Input: part model. Units: mm. Frame: model coordinates. Face numbers are marked on the shaded views. A direction names the side the tool comes from. Round coordinates to 2 decimals unless told otherwise and drop trailing zeros. Order: outer loops, then holes, each group sorted by start corner. A loop starts at its lowest first (then second) coordinate and runs counter-clockwise, first axis right, second up. Notation, with made-up numbers: (72.25, 59.25) -> (117.25, 59.25) arc R26 ccw to (117.25, 81.25) -> close; hole circle Ø9 at (45.5, -36.5). An arc over 180 degrees is marked (long way). Use a Markdown table: item, result.
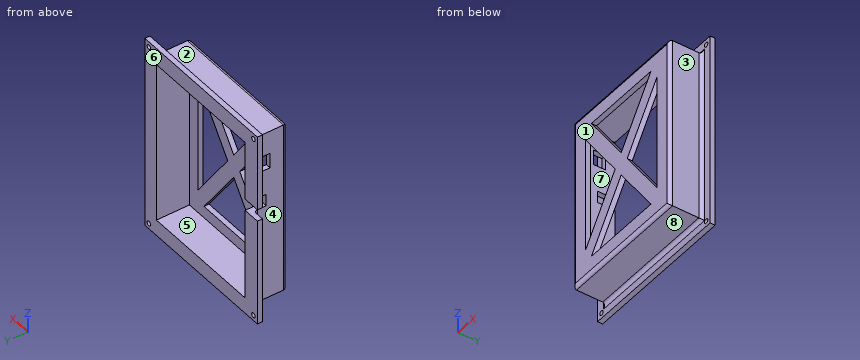
from build123d import *

# Parameters (mm, degrees)
SKETCH1_W              = 72.5
SKETCH1_H              = 96.5
BRACKETBASE_DEPTH      = 3
SKETCH3_W              = 78.5
SKETCH3_H              = 102.5
SKETCH3_W_2            = 72.5
SKETCH3_H_2            = 96.5
BRACKETWALLS_DEPTH     = 22.5
SKETCH4_W              = 7
SKETCH4_H              = 19.5
WIREHOLE_DEPTH         = 22.5
BRACKETFLANGE_DEPTH    = 3
SKETCH7_R              = 1.375
MOUNTINGHOLES_DEPTH    = 4
SKETCH8_W              = 9
SKETCH8_H              = 7
SWITCHHOLE_DEPTH       = 10
BOSS_EXTRUDE1_REACH    = 72.85
SKETCH10_W             = 2.5
SKETCH10_H             = 7
BOSS_EXTRUDE2_DEPTH    = 12.25
FILLET1_R              = 2
FILLET2_R              = 2
SKETCH11_W             = 7
SKETCH11_H             = 10.25
CUT_EXTRUDE1_DEPTH     = 10
WEIGHTREDUCTION1_DEPTH = 23.5


with BuildPart() as part:
    # Sketch1 → bracketBase (new body)
    with BuildSketch(Plane(origin=(0, 0, 0), x_dir=(1, 0, 0), z_dir=(0, 1, 0))):
        with Locations((36.25, 48.25)):
            Rectangle(SKETCH1_W, SKETCH1_H)
    extrude(amount=BRACKETBASE_DEPTH)

    # Sketch3 → bracketWalls (add)
    with BuildSketch(Plane.XZ):
        with Locations((36.25, -48.25)):
            Rectangle(SKETCH3_W, SKETCH3_H)
        with Locations((36.25, -48.25)):
            Rectangle(SKETCH3_W_2, SKETCH3_H_2, mode=Mode.SUBTRACT)
    extrude(amount=-BRACKETWALLS_DEPTH)

    # Sketch4 → wireHole (cut)
    with BuildSketch(Plane.ZY.offset(-72.5)):
        with Locations((-38.65, 12.75)):
            Rectangle(SKETCH4_W, SKETCH4_H)
    wirehole = extrude(amount=-WIREHOLE_DEPTH, mode=Mode.SUBTRACT)

    # Sketch6 → bracketFlange (add)
    with BuildSketch(Plane(origin=(0, 22.5, 0), x_dir=(1, 0, 0), z_dir=(0, 1, 0))):
        Polygon((72.5, 96.5), (72.5, 42.15), (82, 42.15), (82, 106), (-10, 106), (-10, -10), (82, -10), (82, 35.15), (72.5, 35.15), (72.5, 0), (0, 0), (0, 96.5), align=None)
    extrude(amount=-BRACKETFLANGE_DEPTH)

    # Sketch7 → mountingHoles (cut, through all)
    with BuildSketch(Plane.XZ.offset(-19.5)):
        with Locations((78.75, -102.75)):
            Circle(SKETCH7_R)
        with Locations((78.75, 6.75)):
            Circle(SKETCH7_R)
        with Locations((-6.75, -102.75)):
            Circle(SKETCH7_R)
        with Locations((-6.75, 6.75)):
            Circle(SKETCH7_R)
    extrude(amount=-MOUNTINGHOLES_DEPTH, mode=Mode.SUBTRACT)

    # Mirror1: wireHole across plane
    add(wirehole.mirror(Plane(origin=(36, 0, 0), x_dir=(0, 0, 1), z_dir=(1, 0, 0))), mode=Mode.SUBTRACT)

    # Sketch8 → switchHole (cut)
    with BuildSketch(Plane.ZY.offset(3)):
        with Locations((-15.23, 13.5)):
            Rectangle(SKETCH8_W, SKETCH8_H)
    extrude(amount=-SWITCHHOLE_DEPTH, mode=Mode.SUBTRACT)

    # Sketch9 → Boss-Extrude1 (add, up to next)
    with BuildSketch(Plane(origin=(0, 0, -35.15), x_dir=(-1, 0, 0), z_dir=(0, 0, -1)), mode=Mode.PRIVATE) as boss_extrude1_sk1:
        Polygon((-72.5, 3), (-72.5, 22.5), (-82, 22.5), (-82, 19.5), (-75.5, 19.5), (-75.5, 3), align=None)
    boss_extrude1_tool1 = extrude(boss_extrude1_sk1.sketch, amount=BOSS_EXTRUDE1_REACH, mode=Mode.PRIVATE) - part.part
    add(boss_extrude1_tool1.solids().sort_by_distance((75.1875, 14.8125, -35.15))[0])

    # Sketch10 → Boss-Extrude2 (add)
    with BuildSketch(Plane.XZ):
        with Locations((-1.75, -38.65)):
            Rectangle(SKETCH10_W, SKETCH10_H)
    extrude(amount=-BOSS_EXTRUDE2_DEPTH)

    # Fillet1
    fillet1_edges = [part.edges().sort_by_distance(p)[0] for p in [
        (-3, 19.5, -16.075),
        (36.25, 19.5, 3),
        (75.5, 19.5, -48.25),
        (36.25, 19.5, -99.5),
        (-3, 19.5, -70.825),
    ]]
    fillet(fillet1_edges, radius=FILLET1_R)

    # Fillet2
    fillet2_edges = [part.edges().sort_by_distance(p)[0] for p in [
        (36.25, 0, 3),
        (-3, 0, -48.25),
        (36.25, 0, -99.5),
        (75.5, 0, -48.25),
    ]]
    fillet(fillet2_edges, radius=FILLET2_R)

    # Sketch11 → Cut-Extrude1 (cut)
    with BuildSketch(Plane.ZY.offset(0.5)):
        with Locations((-38.65, 17.375)):
            Rectangle(SKETCH11_W, SKETCH11_H)
    extrude(amount=-CUT_EXTRUDE1_DEPTH, mode=Mode.SUBTRACT)

    # Sketch12 → weightReduction1 (cut, through all)
    with BuildSketch(Plane.XZ):
        Polygon((11.903565914, -89.5), (36.25, -55.165285264), (60.596434086, -89.5), align=None)
        Polygon((65.5, -82.584714736), (41.153565914, -48.25), (65.5, -13.915285264), align=None)
        Polygon((60.596434086, -7), (11.903565914, -7), (36.25, -41.334714736), align=None)
        Polygon((7, -13.915285264), (7, -82.584714736), (31.346434086, -48.25), align=None)
    extrude(amount=-WEIGHTREDUCTION1_DEPTH, mode=Mode.SUBTRACT)


solid = part.part
1) Cut plane D-D on z = 6.75. Return loops of the section in (x, y) (3 decimals).
Answer key:
| item | result |
|---|---|
| outline | (-10, 19.5) -> (-8.125, 19.5) -> (-8.125, 22.5) -> (-10, 22.5) -> close; (-5.375, 19.5) -> (77.375, 19.5) -> (77.375, 22.5) -> (-5.375, 22.5) -> close; (80.125, 19.5) -> (82, 19.5) -> (82, 22.5) -> (80.125, 22.5) -> close |
2) Draft query along Z for the marked faces 6, 7 and 8. Return one class per face: released by +Z, released by -Z, zero draft, split by the parting line, or undercut.
Answer key:
| item | result |
|---|---|
| face 6 | zero draft |
| face 7 | undercut |
| face 8 | released by -Z |
3) Cut plane B-B on y = 4.5. Return loops of the section in (x, z).
Answer key:
| item | result |
|---|---|
| outline | (-3, -99.5) -> (75.5, -99.5) -> (75.5, 3) -> (-3, 3) -> close; hole (0, -96.5) -> (72.5, -96.5) -> (72.5, 0) -> (0, 0) -> close |
4) Set-up query: the marked faces 1, 2, 3, 4 and 5. Return all of +Z, -Z, +X, -X, +Y, -Y with unobstructed straight access to the full face (end or side cutting, diameter ignored); none if empty.
Answer key:
| item | result |
|---|---|
| face 1 | +Z, -Z, +X, -X, -Y |
| face 2 | +Z, +X, -X, -Y |
| face 3 | +Z, -Z, +X, -Y |
| face 4 | +Z, -Z, -X, -Y |
| face 5 | +Y |
5) Ray query, probe 1 along Z at (x, y) = (78.75, 21.85) (3 decimals); probe 2 along Z at (x, y) = (-6.75, 21.3) (3 decimals); probe 3 along X at (y, z) = (12.75, -4). Return the intervals inside material, ascending.
Answer key:
| item | result |
|---|---|
| probe 1 | z = -106 to -104.125, -101.375 to 5.375, 8.125 to 10 |
| probe 2 | z = -106 to -104.125, -101.375 to -42.15, -35.15 to 5.375, 8.125 to 10 |
| probe 3 | x = -3 to 0, 72.5 to 75.5 |
6) Cut plane C-C on x = -6.75. Return loops of the section in (y, z) (3 decimals), and give its area (4 significant figures).
Answer key:
| item | result |
|---|---|
| outline | (19.5, -106) -> (22.5, -106) -> (22.5, -104.125) -> (19.5, -104.125) -> close; (19.5, -101.375) -> (22.5, -101.375) -> (22.5, -42.15) -> (19.5, -42.15) -> close; (19.5, -35.15) -> (22.5, -35.15) -> (22.5, 5.375) -> (19.5, 5.375) -> close; (19.5, 8.125) -> (22.5, 8.125) -> (22.5, 10) -> (19.5, 10) -> close |
| area | 310.5 mm^2 |
7) Cut plane A-A on x = 78.75. Return loops of the section in (y, z) (3 decimals).
Answer key:
| item | result |
|---|---|
| outline | (19.5, -106) -> (22.5, -106) -> (22.5, -104.125) -> (19.5, -104.125) -> close; (19.5, -101.375) -> (22.5, -101.375) -> (22.5, 5.375) -> (19.5, 5.375) -> close; (19.5, 8.125) -> (22.5, 8.125) -> (22.5, 10) -> (19.5, 10) -> close |
8) Contact query for flat-ended pins moving along their axis: P1, Ø2, axis at x = 41, y = 10, coming from the -Z side; P2, Ø2.5, axis at x = -2, y = 13, coming from the +Z side; P3, Ø8, axis at y = 8.5, z = -51, coming from the -X side; P4, Ø0.9, axis at x = -1.5, z = -16, coming from the -Y side. Output: stop coordinate, or through.
Answer key:
| item | result |
|---|---|
| P1 | stops at z = -99.5 |
| P2 | stops at z = 3 |
| P3 | stops at x = -3 |
| P4 | stops at y = 0 |
